Verification items for the finished model (mm, model axes). Coordinates: 2 decimals unless noted, no trailing zeros. Loops run counter-clockwise (first coordinate to the right, second up) from the corner with the lowest first, then second, coordinate; pieces in that order, holes last. Notation, with made-up numbers: (-33, 2.5) -> (17, 2.5) arc R15 ccw to (17, 18.5) -> close; hole circle Ø10 at (67, 89). An arc over 180 degrees is marked (long way). Write item = value, one per line.
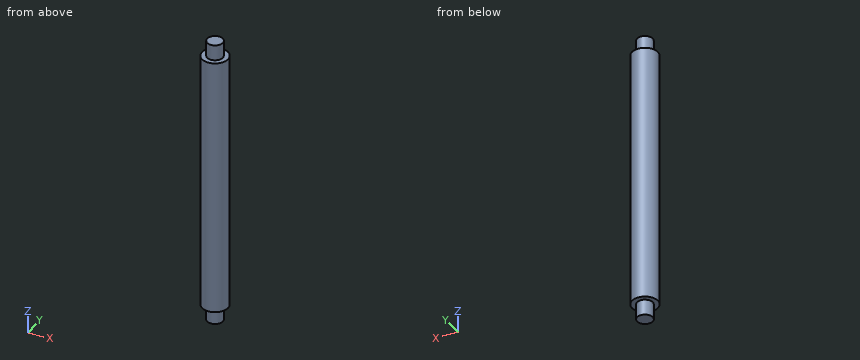
Autodesk Inventor part; units mm, degrees
ref_plane "YZ Plane" through (0, 0, 0) normal (1, 0, 0) x (0, 1, 0)
ref_plane "XZ Plane" through (0, 0, 0) normal (0, 1, 0) x (-1, 0, 0)
ref_plane "XY Plane" through (0, 0, 0) normal (0, 0, 1) x (1, 0, 0)
sketch "Sketch1" plane through (0, 0, 0) normal (0, 0, 1) x (1, 0, 0)
  circle A0 centre (0, 0) radius 2.5
  dimension "d0" = 5
extrude "Extrusion1" add sketch "Sketch1" along normal blind 50
sketch "Sketch2" plane through (0, 0, 50) normal (0, 0, 1) x (1, 0, 0)
  circle A0 centre (0, 0) radius 2.5
  circle A1 centre (0, 0) radius 1.5
  dimension "d3" = 3
extrude "Extrusion2" add sketch "Sketch2" along normal blind 3 contours A1
thread "Thread1"
sketch "Sketch3" plane through (0, 0, 0) normal (0, 0, -1) x (-1, 0, 0)
  circle A0 centre (0, 0) radius 2.5
  circle A1 centre (0, 0) radius 1.5
  dimension "d8" = 3
extrude "Extrusion3" add sketch "Sketch3" along normal blind 3 contours A1
thread "Thread2"
properties part number "spacer 4 cm"
1) Material ranges on line 1 (Z direction, x = -1.95, y = -0.5); line 2 (X direction, y = -0.1, z = 8.5), recorded low to high.
Ans:
line_1 = 0 to 50
line_2 = -2.5 to 2.5
2) Sectioned sample at A-A, the plane y = 0. Record the cut outline in (x, z), plus the area to 3 significant figures.
Ans:
outline = (-2.5, 0) -> (-1.5, 0) -> (-1.5, -3) -> (1.5, -3) -> (1.5, 0) -> (2.5, 0) -> (2.5, 50) -> (1.5, 50) -> (1.5, 53) -> (-1.5, 53) -> (-1.5, 50) -> (-2.5, 50) -> close
area = 268 mm2
3) Sectioned sample at C-C, the plane z = 6. Record the cut outline in (x, y), plus the area to 3 significant figures.
Ans:
outline = circle Ø5 at (0, 0)
area = 19.6 mm2
4) Depth check by flat-ended pin: pin 1 Ø2 at (y, z) = (-1.5, 7.5) entering from +X. Enter the tip coordinate at first touch or a pass-through.
Ans:
pin_1 = 2.45
5) Sectioned sample at D-D, the plane x = 2. Record the cut outline in (y, z), plus the area to 3 significant figures.
Ans:
outline = (-1.5, 0) -> (1.5, 0) -> (1.5, 50) -> (-1.5, 50) -> close
area = 150 mm2
